Verification items for the finished model (mm, model axes). Face numbers are marked on the shaded views. A direction names the side the tool comes from. Round coordinates to 2 decimals unless told otherwise and drop trailing zeros. Loops run counter-clockwise (first coordinate to the right, second up) from the corner with the lowest first, then second, coordinate; pieces in that order, holes last. Notation, with made-up numbers: (3, -30.5) -> (60, -30.5) arc R19 cw to (60, -24.5) -> close; hole circle Ø7 at (30.5, -14). An arc over 180 degrees is marked (long way). Use a Markdown table: item, result. Add a question column.
```python
from build123d import *

# Parameters (mm, degrees)
SKETCH012_W     = 17
SKETCH012_H     = 21
PAD009_DEPTH    = 29
SKETCH013_W     = 13.1
SKETCH013_H     = 17
POCKET001_DEPTH = 23.7
SKETCH014_W     = 11.5
SKETCH014_H     = 1.2
SKETCH014_W_2   = 3.205285
SKETCH014_H_2   = 1.736194
POCKET002_DEPTH = 26.5
SKETCH016_R     = 0.6
POCKET003_DEPTH = 27


with BuildPart() as part:
    # Sketch012 → Pad009 (new body)
    with BuildSketch(Plane.XZ):
        with Locations((1.5, -2)):
            Rectangle(SKETCH012_W, SKETCH012_H)
    extrude(amount=PAD009_DEPTH)

    # Sketch013 (on Face5 of Pad009) → Pocket001 (cut)
    with BuildSketch(Plane(origin=(0, 0, 0), x_dir=(1, 0, 0), z_dir=(0, 1, 0))):
        with Locations((2.05, 2)):
            Rectangle(SKETCH013_W, SKETCH013_H)
    extrude(amount=-POCKET001_DEPTH, mode=Mode.SUBTRACT)

    # Sketch014 (on Face4 of Pocket001) → Pocket002 (cut)
    with BuildSketch(Plane(origin=(0, 0, 0), x_dir=(1, 0, 0), z_dir=(0, 1, 0))):
        Rectangle(SKETCH014_W, SKETCH014_H)
        with Locations((9.189982, -4.640042)):
            Rectangle(SKETCH014_W_2, SKETCH014_H_2)
    extrude(amount=-POCKET002_DEPTH, mode=Mode.SUBTRACT)

    # Sketch016 (on Face6 of Pocket002) → Pocket003 (cut)
    with BuildSketch(Plane(origin=(0, 0, -12.5), x_dir=(1, 0, 0), z_dir=(0, 0, -1))):
        with Locations((0, 3)):
            Circle(SKETCH016_R)
    extrude(amount=-POCKET003_DEPTH, mode=Mode.SUBTRACT)


solid = part.part
```
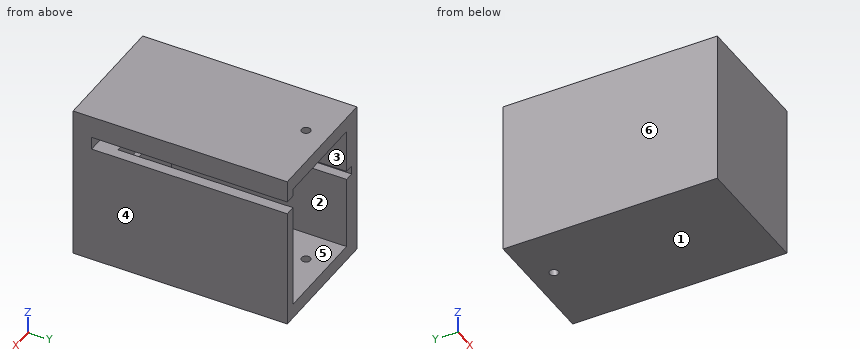
1) Sectioned sample at C-C on x = 4. Enter the section's corners in (y, z).
2) Access from +Z, -Z, +X, -X, +Y, -Y to the whole of each face (thin tool, end or side, straight path). Record for the marked faces 5 and 6.
3) Release check for a two-part mould opening along X. For the marked faces 1, 2, 3 and 4 record: released by +X, released by -X, zero draft, split by the parting line, or undercut.
4) Sectioned sample at D-D on z = -2.25. Enter the section's corners in (x, y).
5) Go/stop test with flat-tipped pins: pin 1 (1 mm diameter, centred on x = -1, z = 0, fed in from +Y); pin 2 (1 mm diameter, centred on x = 3.5, z = 0.5, fed in from +Y). Record where each tip stops, or that it passes through.
6) Sectioned sample at B-B on x = 0. Enter the section's corners in (y, z), then the cut area to 3 significant figures.
7) Sectioned sample at A-A on y = -3. Enter the section's corners in (x, z), then the cut area to 3 significant figures.
8) Thickness scan on line 1 (X direction, y = -18, z = -3.5); line 2 (X direction, y = -3, z = 7.65); line 3 (Z direction, x = 0, y = -8.5). Record the ranges inside material, lowest first.
Geometry results:
| question | item | result |
|---|---|---|
| 1 | outline | (-29, -12.5) -> (0, -12.5) -> (0, -10.5) -> (-23.7, -10.5) -> (-23.7, -0.6) -> (-26.5, -0.6) -> (-26.5, 0.6) -> (-23.7, 0.6) -> (-23.7, 6.5) -> (0, 6.5) -> (0, 8.5) -> (-29, 8.5) -> close |
| 2 | face 5 | +Y |
| 2 | face 6 | +Z, -Z, -X, +Y, -Y |
| 3 | face 1 | zero draft |
| 3 | face 2 | undercut |
| 3 | face 3 | undercut |
| 3 | face 4 | released by +X |
| 4 | outline | (-7, -29) -> (10, -29) -> (10, 0) -> (8.6, 0) -> (8.6, -23.7) -> (-4.5, -23.7) -> (-4.5, 0) -> (-7, 0) -> close |
| 5 | pin 1 | y = -26.5 |
| 5 | pin 2 | y = -23.7 |
| 6 | outline | (-29, -12.5) -> (-3.6, -12.5) -> (-3.6, -10.5) -> (-23.7, -10.5) -> (-23.7, -0.6) -> (-26.5, -0.6) -> (-26.5, 0.6) -> (-23.7, 0.6) -> (-23.7, 6.5) -> (-3.6, 6.5) -> (-3.6, 8.5) -> (-29, 8.5) -> close; (-2.4, -12.5) -> (0, -12.5) -> (0, -10.5) -> (-2.4, -10.5) -> close; (-2.4, 6.5) -> (0, 6.5) -> (0, 8.5) -> (-2.4, 8.5) -> close |
| 6 | area | 198 mm^2 |
| 7 | outline | (-7, -12.5) -> (-0.6, -12.5) -> (-0.6, -10.5) -> (-4.5, -10.5) -> (-4.5, -0.6) -> (-5.75, -0.6) -> (-5.75, 0.6) -> (-4.5, 0.6) -> (-4.5, 6.5) -> (-0.6, 6.5) -> (-0.6, 8.5) -> (-7, 8.5) -> close; (0.6, -12.5) -> (10, -12.5) -> (10, 3.77) -> (8.6, 3.77) -> (8.6, -10.5) -> (0.6, -10.5) -> close; (0.6, 6.5) -> (8.6, 6.5) -> (8.6, 5.51) -> (10, 5.51) -> (10, 8.5) -> (0.6, 8.5) -> close |
| 7 | area | 126 mm^2 |
| 8 | line 1 | -7 to -4.5, 8.6 to 10 |
| 8 | line 2 | -7 to -0.6, 0.6 to 10 |
| 8 | line 3 | -12.5 to -10.5, 6.5 to 8.5 |
